from build123d import *

# Parameters (mm, degrees)
SKETCH1_R           = 12.5
BOSS_EXTRUDE1_DEPTH = 3
SKETCH2_R           = 4
BOSS_EXTRUDE2_DEPTH = 5
SKETCH5_R           = 2
CUT_EXTRUDE3_DEPTH  = 8
SKETCH4_R           = 1
CUT_EXTRUDE4_DEPTH  = 8
SKETCH3_R           = 1
CUT_EXTRUDE7_DEPTH  = 3
SKETCH11_R          = 1.073090014
SKETCH11_R_2        = 1
CUT_EXTRUDE9_DEPTH  = 3


with BuildPart() as part:
    # Sketch1 → Boss-Extrude1 (new body)
    with BuildSketch(Plane(origin=(0, 0, 0), x_dir=(1, 0, 0), z_dir=(0, 1, 0))):
        Circle(SKETCH1_R)
    extrude(amount=BOSS_EXTRUDE1_DEPTH)

    # Sketch2 → Boss-Extrude2 (add)
    with BuildSketch(Plane(origin=(0, 0, 0), x_dir=(1, 0, 0), z_dir=(0, 1, 0))):
        Circle(SKETCH2_R)
    extrude(amount=BOSS_EXTRUDE2_DEPTH)

    # Sketch5 → Cut-Extrude3 (cut)
    with BuildSketch(Plane(origin=(0, 5, 0), x_dir=(1, 0, 0), z_dir=(0, 1, 0))):
        Circle(SKETCH5_R)
    extrude(amount=-CUT_EXTRUDE3_DEPTH, mode=Mode.SUBTRACT)

    # Sketch4 → Cut-Extrude4 (cut)
    with BuildSketch(Plane(origin=(0, 3, 0), x_dir=(1, 0, 0), z_dir=(0, 1, 0))):
        with Locations((5.080770429, 8.613345791)):
            Circle(SKETCH4_R)
    extrude(amount=-CUT_EXTRUDE4_DEPTH, mode=Mode.SUBTRACT)

    # Sketch3 → Cut-Extrude7 (cut)
    with BuildSketch(Plane(origin=(0, 0, 0), x_dir=(1, 0, 0), z_dir=(0, 1, 0))):
        with Locations((-5.080770429, -8.613345791)):
            Circle(SKETCH3_R)
    extrude(amount=CUT_EXTRUDE7_DEPTH, mode=Mode.SUBTRACT)

    # Sketch11 → Cut-Extrude9 (cut)
    with BuildSketch(Plane(origin=(0, 3, 0), x_dir=(1, 0, 0), z_dir=(0, 1, 0))):
        with Locations((-4.754881291, 8.797221374)):
            Circle(SKETCH11_R)
        with Locations((-9.996057838, 0.280762697)):
            Circle(SKETCH11_R_2)
        with Locations((4.754881291, -8.797221374)):
            Circle(SKETCH11_R_2)
        with Locations((9.996057838, -0.280762697)):
            Circle(SKETCH11_R_2)
    extrude(amount=-CUT_EXTRUDE9_DEPTH, mode=Mode.SUBTRACT)


solid = part.part
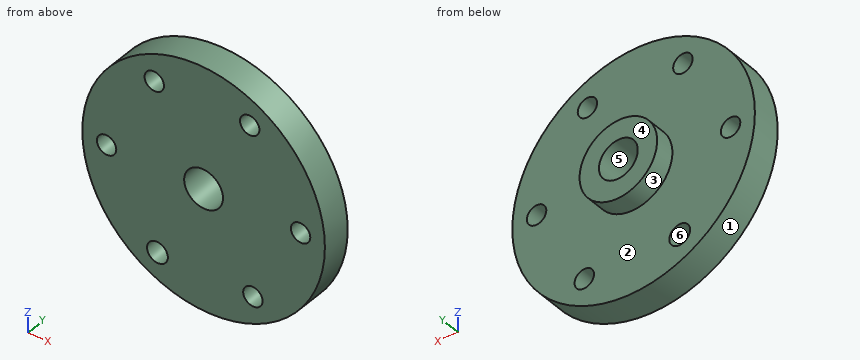
Geometry: final body of the model. Coordinates: model frame, mm. Face numbers are marked on the shaded views. A direction names the side the tool comes from. Give positions to 0.01 mm unless a question says otherwise; leave off trailing zeros. Write each loop counter-clockwise with the first axis right and the second up, starting at its lowest first coordinate (ties: lowest second). Pieces come first, ordered by that corner, then holes.
(1) Access query for the marked faces 1 and 2. Directions: +Z, -Z, +X, -X, +Y, -Y. A direction counts if a zero-diameter tool reaches every point of the face in a straight line with its end or side. Return the directions, or none.
(2) Cut plane B-B, the plane y = 3.5. Return loops of the section in (x, z).
(3) Cut plane A-A, the plane x = 0. Return loops of the section in (y, z).
(4) Ray query, line 1 (Z direction, x = 0, y = 4.05); line 2 (Z direction, x = 0, y = 2.55); line 3 (Z direction, x = -5.5, y = 2.1) (3 decimals). Return the intervals inside material, ascending.
(5) First-contact query: P1, Ø3, axis at y = 2, z = 6, coming from the -X side; P2, Ø3, axis at x = 3.5, y = 2.5, coming from the -Z side; P3, Ø3, axis at x = -4.75, z = -8.8, coming from the +Y side. Flat tips, straight axial feed; report the tip coordinate or a pass-through.
(6) Cut plane C-C, the plane x = -10.5. Return loops of the section in (y, z), then the cut area to 3 significant figures.
(7) Mould query, pull axis X, two halves, no side actions, for the marked faces 3, 4, 5 and 6. Classes: released by +X, released by -X, zero draft, split by the parting line, or undercut.
(8) Cut plane D-D, the plane y = 0.6. Return loops of the section in (x, z), then the cut area to 3 significant figures.
Values follow:
1. face 1: +Y, -Y
1. face 2: +Y
2. outline: circle Ø8 at (0, 0); hole circle Ø4 at (0, 0)
3. outline: (0, -12.5) - (3, -12.5) - (3, -4) - (5, -4) - (5, -2) - (0, -2) - close; (0, 2) - (5, 2) - (5, 4) - (3, 4) - (3, 12.5) - (0, 12.5) - close
4. line 1: z = -4 to -2, 2 to 4
4. line 2: z = -12.5 to -2, 2 to 12.5
4. line 3: z = -11.225 to -9.569, -8.025 to 7.705, 9.521 to 11.225
5. P1: stops at x = -11.66
5. P2: stops at z = -12.34
5. P3: stops at y = 3
6. outline: (0, -6.78) - (3, -6.78) - (3, -1.14) - (0, -1.14) - close; (0, 0.58) - (3, 0.58) - (3, 6.78) - (0, 6.78) - close
6. area: 35.5 mm2
7. face 3: split by the parting line
7. face 4: zero draft
7. face 5: undercut
7. face 6: undercut
8. outline: circle Ø25 at (0, 0); hole circle Ø2 at (-10, -0.28); hole circle Ø2 at (-5.08, 8.61); hole circle Ø2.15 at (-4.75, -8.8); hole circle Ø4 at (0, 0); hole circle Ø2 at (4.75, 8.8); hole circle Ø2 at (5.08, -8.61); hole circle Ø2 at (10, 0.28)
8. area: 459 mm2
